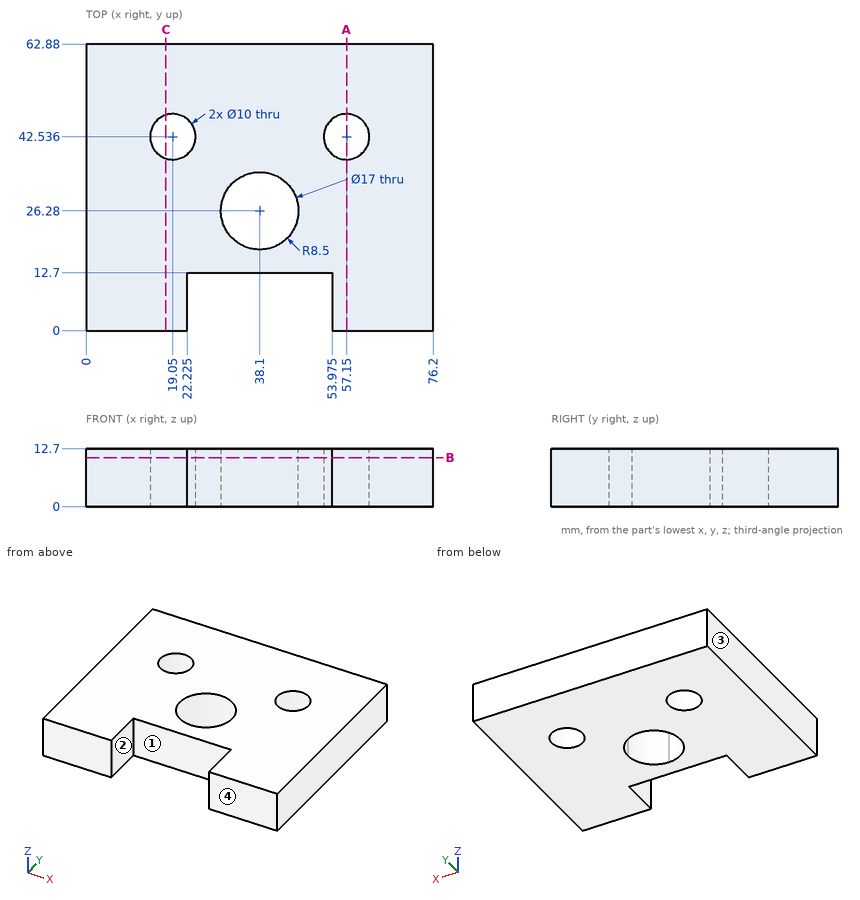
Job drawing, mm, ordinate dimensions from the low corner. One solid piece. Coordinates: 2 decimals unless noted, no trailing zeros. Order: outer loops, then holes, each group sorted by start corner. A loop starts at its lowest first (then second) coordinate and runs counter-clockwise, first axis right, second up. Notation, with made-up numbers: (28, -2) -> (75, -2) arc R31 ccw to (75, 37) -> close; hole circle Ø6 at (76, -3). An arc over 180 degrees is marked (long way). Answer in a Markdown table with one row per item. Add a question column.
Q1. Wall check: line 1 along Y through (x, z) = (19.05, 9.25); line 2 along X through (y, z) = (9, 9.5) (1 decimal); line 3 along X through (y, z) = (26.28, 9.5). Give the ranges that are in metal, low to high. Write a range as [from, to].
Q2. Drop a flat-ended pin along its axis: pin 1 (6 mm diameter, centred on x = 34, z = 2, fed in from -Y). Give the stop position or say it passes through.
Q3. Band-saw the part on C-C, the plane x = 17.5. List the corners of the cut face in (y, z).
Q4. Band-saw the part on B-B, the plane z = 10.75. Give the number of separate pieces and of enclosed holes in the cut face, then the cut area to 3 significant figures.
Q5. Band-saw the part on A-A, the plane x = 57.15. List the corners of the cut face in (y, z).
Q6. Mould opens along X. For the marked faces 1, 2, 3 and 4 say: +X half, -X half, draft (parallel to the pull), parting line (faces both ways), or undercut.
Answers follow:
| question | item | result |
|---|---|---|
| 1 | line 1 | [0, 37.54], [47.54, 62.88] |
| 1 | line 2 | [0, 22.2], [54, 76.2] |
| 1 | line 3 | [0, 29.6], [46.6, 76.2] |
| 2 | pin 1 | y = 12.7 |
| 3 | outline | (0, 0) -> (37.78, 0) -> (37.78, 12.7) -> (0, 12.7) -> close; (47.29, 0) -> (62.88, 0) -> (62.88, 12.7) -> (47.29, 12.7) -> close |
| 4 | separate pieces | 1 |
| 4 | enclosed holes | 3 |
| 4 | area | 4,000 mm^2 |
| 5 | outline | (0, 0) -> (37.54, 0) -> (37.54, 12.7) -> (0, 12.7) -> close; (47.54, 0) -> (62.88, 0) -> (62.88, 12.7) -> (47.54, 12.7) -> close |
| 6 | face 1 | undercut |
| 6 | face 2 | undercut |
| 6 | face 3 | -X half |
| 6 | face 4 | draft |
